Check sheet for the modelled part. Datum: model origin and axes. Units: mm. Face numbers are marked on the shaded views. Round coordinates to 2 decimals unless told otherwise and drop trailing zeros. Loops run counter-clockwise (first coordinate to the right, second up) from the corner with the lowest first, then second, coordinate; pieces in that order, holes last. Notation, with made-up numbers: (-30.75, -26.75) - (-14.75, -26.75) arc R21 ccw to (-14.75, 4.25) - close; hole circle Ø4 at (87.25, 53.25). An arc over 180 degrees is marked (long way). Put each result on its own line as item: value. Start each with the question number.
Item 1: Draft check along Y on the marked faces 1, 2 and 3. Enter one of: pulls with the +Y half, pulls with the -Y half, needs draft (parallel to the pull), parting line crosses it, or undercut.
Item 2: Material ranges on line 1 along Z through (x, y) = (1.25, -2.25); line 2 along Y through (x, z) = (-4.5, 7.5); line 3 along Z through (x, y) = (-2, -0.5), recorded low to high.
Item 3: Section check A-A, the plane y = -2.25. Record the cut outline in (x, z).
Item 4: Gauge pin test, flat ends, axial feed: pin 1 Ø3 at (x, y) = (4, 0.5) entering from -Z; pin 2 Ø1.5 at (x, y) = (-2.5, 1) entering from -Z. Record the tip position at first contact, or that the pin passes through.
Autodesk Inventor part; units mm, degrees
ref_plane "YZ Plane" through (0, 0, 0) normal (1, 0, 0) x (0, 1, 0)
ref_plane "XZ Plane" through (0, 0, 0) normal (0, 1, 0) x (-1, 0, 0)
ref_plane "XY Plane" through (0, 0, 0) normal (0, 0, 1) x (1, 0, 0)
sketch "Sketch1" plane through (0, 0, 0) normal (0, 0, 1) x (1, 0, 0)
  line L0 (-5, 4) -> (5, 4)
  line L1 (5, 4) -> (5, -4)
  line L2 (5, -4) -> (-5, -4)
  line L3 (-5, -4) -> (-5, 4)
  line L4 (-7, 0) -> (7, 0) construction
  line L5 (0, -5.6) -> (0, 5.6) construction
  point P0 (0, 0)
  point P1 (0, -4)
  point P2 (-5, 0)
  dimension "d0" = 10
  dimension "d1" = 8
extrude "Extrusion1" add sketch "Sketch1" along normal blind 32
fillet "Fillet3" radius 4 4 edges at (5, 0, 32) (-5, 0, 32) (5, 0, 0) (-5, 0, 0)
fillet "Fillet1" radius 0.6 4 edges at (-5, 4, 16) (-5, -4, 16) (5, 4, 16) (5, -4, 16)
equation "\"d2\" = GearKey_L"
equation "\"TD\" = 0.3"
equation "\"Ball_DIA\" = 6"
equation "\"Screw_L\" = 292"
equation "\"Screw_DIA\" = 36"
equation "\"Nut_OD\" = 66"
equation "\"BPath_REVQ\" = 5.75"
equation "\"Tread_OFFSET\" = 8.075"
equation "\"SteeringColumn_DIA\" = 26"
equation "\"SteeringColumnChamfer_DEG\" = 20deg"
equation "\"Rack_L\" = 307.252"
equation "\"NutCapTread_L\" = 25"
equation "\"NutCapTread_THICKNESS\" = 5.365"
equation "\"SupportFlange_THICKNESS\" = 5"
equation "\"GearKey_L\" = 32"
properties part number "MCEN4000:G1K" material "STEEL, AISI 1015"
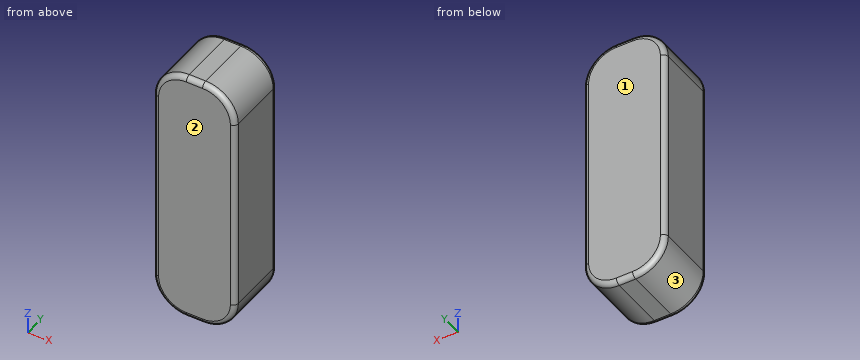
Check result:
1. face 1: pulls with the +Y half
1. face 2: pulls with the -Y half
1. face 3: needs draft
2. line 1: 0.01 to 31.99
2. line 2: -3.99 to 3.99
2. line 3: 0.13 to 31.87
3. outline: (-5, 4) arc R4 ccw to (-1, 0) - (1, 0) arc R4 ccw to (5, 4) - (5, 28) arc R4 ccw to (1, 32) - (-1, 32) arc R4 ccw to (-5, 28) - close
4. pin 1: z = 0.29
4. pin 2: z = 0.07
